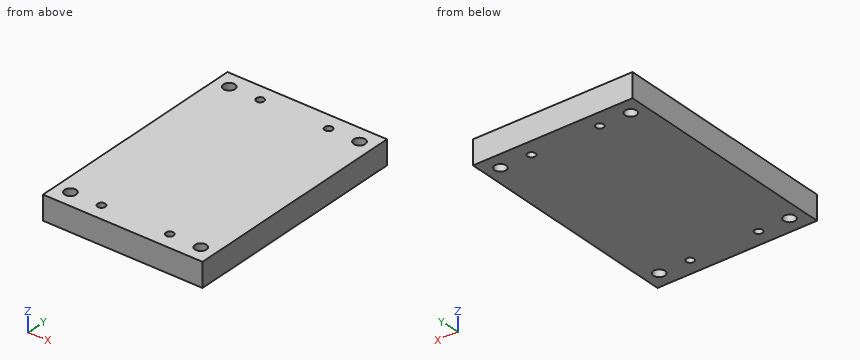
```python
from build123d import *

# Parameters (mm, degrees)
F0_W     = 60.96
F0_H     = 6.35
F1_DEPTH = 21
F2_R     = 1.016
F3_R     = 1.516992
F4_DEPTH = 6.35


with BuildPart() as f1:
    # F0 (on Right) → F1 (new body, symmetric)
    with BuildSketch(Plane.YZ):
        Rectangle(F0_W, F0_H)
    extrude(amount=F1_DEPTH, both=True)

    # F2 (on face) + F3 (on face) → F4 (cut, through all)
    with BuildSketch(Plane.XY.offset(3.175)):
        with Locations((-9, -26.23)):
            Circle(F2_R)
        with Locations((9, -26.23)):
            Circle(F2_R)
        with Locations((9, 26.23)):
            Circle(F2_R)
        with Locations((-9, 26.23)):
            Circle(F2_R)
    with BuildSketch(Plane.XY.offset(3.175)):
        with Locations((-17.153514, 26.2382)):
            Circle(F3_R)
        with Locations((17.153514, 26.2382)):
            Circle(F3_R)
        with Locations((17.153514, -26.2382)):
            Circle(F3_R)
        with Locations((-17.153514, -26.2382)):
            Circle(F3_R)
    extrude(amount=-F4_DEPTH, mode=Mode.SUBTRACT)


solid = f1.part
```
The model under review builds one solid part; all positions refer to its coordinate system, in mm. Give positions to 0.01 mm unless a question says otherwise; leave off trailing zeros. Write each loop counter-clockwise with the first axis right and the second up, starting at its lowest first coordinate (ties: lowest second). Pieces come first, ordered by that corner, then holes. Notation, with made-up numbers: (50.25, -22.5) - (82.25, -22.5) arc R20 ccw to (82.25, 13.5) - close; hole circle Ø8 at (64, 79). An arc over 180 degrees is marked (long way). Answer in a Markdown table with one row per item. Add a question column.
1. We need section B-B on z = 0. State how many separate pieces and enclosed holes the cut face has, then the cut area to 3 significant figures.
2. Wall thickness on line 1 along Y through (x, z) = (-17.5, -0.5); line 2 along Y through (x, z) = (9.5, 2.5); line 3 along X through (y, z) = (27.5, -1.75): over which ranges is each line inside the solid? List them lowest first. Write a range as [from, to].
3. We need section A-A on x = -9. Write out the cut boundary in (y, z) (3 decimals), then the cut area to 3 significant figures.
4. We need section C-C on x = 17.5. Write out the cut boundary in (y, z) (3 decimals), then the cut area to 3 significant figures.
5. Insertion check: P1, Ø2.5, axis at x = 17.15, y = -26.24, coming from the -Z side. The pin has a flat end and moves straight along its axis. Give the tip position at first contact, or say it passes through.
Ans:
| question | item | result |
|---|---|---|
| 1 | separate pieces | 1 |
| 1 | enclosed holes | 8 |
| 1 | area | 2,520 mm^2 |
| 2 | line 1 | y = [-30.48, -27.72], [-24.76, 24.76], [27.72, 30.48] |
| 2 | line 2 | y = [-30.48, -27.11], [-25.35, 25.35], [27.11, 30.48] |
| 2 | line 3 | x = [-21, -18], [-16.31, 16.31], [18, 21] |
| 3 | outline | (-30.48, -3.175) - (-27.246, -3.175) - (-27.246, 3.175) - (-30.48, 3.175) - close; (-25.214, -3.175) - (25.214, -3.175) - (25.214, 3.175) - (-25.214, 3.175) - close; (27.246, -3.175) - (30.48, -3.175) - (30.48, 3.175) - (27.246, 3.175) - close |
| 3 | area | 361 mm^2 |
| 4 | outline | (-30.48, -3.175) - (-27.715, -3.175) - (-27.715, 3.175) - (-30.48, 3.175) - close; (-24.761, -3.175) - (24.761, -3.175) - (24.761, 3.175) - (-24.761, 3.175) - close; (27.715, -3.175) - (30.48, -3.175) - (30.48, 3.175) - (27.715, 3.175) - close |
| 4 | area | 350 mm^2 |
| 5 | P1 | passes through |
